Geometry check sheet. Reference: the model listing, model coordinates, mm. A direction names the side the tool comes from. Coordinates: 2 decimals unless noted, no trailing zeros. Order: outer loops, then holes, each group sorted by start corner. A loop starts at its lowest first (then second) coordinate and runs counter-clockwise, first axis right, second up. Notation, with made-up numbers: (34.5, -20) - (89.5, -20) arc R29 cw to (89.5, 5) - close; hole circle Ø11 at (5.5, -15). An arc over 180 degrees is marked (long way). Put each result on its own line as item: value.
from build123d import *

# Parameters (mm, degrees)
SKETCH1_R           = 5.1
SKETCH1_R_2         = 4.1
BOSS_EXTRUDE1_DEPTH = 5
SKETCH7_R           = 2.6
CUT_EXTRUDE1_DEPTH  = 7
BOSS_EXTRUDE7_DEPTH = 8
SKETCH9_R           = 1.5
CUT_EXTRUDE2_DEPTH  = 7
CUT_EXTRUDE3_DEPTH  = 10
SKETCH11_R          = 1
CUT_EXTRUDE4_DEPTH  = 10
CUT_EXTRUDE5_START  = 5
CUT_EXTRUDE5_DEPTH  = 5


with BuildPart() as part:
    # Sketch1 → Boss-Extrude1 (new body)
    with BuildSketch(Plane.XY):
        with BuildLine():
            Line((-58.265804598, 27.46480771), (50.206034483, 32.957769253))
            ThreePointArc((50.206034483, 32.957769253), (84.875, 0), (50.206034483, -32.957769253))
            Line((50.206034483, -32.957769253), (-58.265804598, -27.46480771))
            ThreePointArc((-58.265804598, -27.46480771), (-61.107119662, -27.172397082), (-63.902777778, -26.586845234))
            Line((-63.902777778, -26.586845234), (-105.963888889, -15.468709954))
            ThreePointArc((-105.963888889, -15.468709954), (-117.875, 0), (-105.963888889, 15.468709954))
            Line((-105.963888889, 15.468709954), (-63.902777778, 26.586845234))
            ThreePointArc((-63.902777778, 26.586845234), (-61.107119662, 27.172397082), (-58.265804598, 27.46480771))
        make_face()
        with Locations((51.875, 0)):
            Circle(SKETCH1_R, mode=Mode.SUBTRACT)
        with Locations((-101.875, 0)):
            Circle(SKETCH1_R_2, mode=Mode.SUBTRACT)
        with BuildLine():
            Line((-46.875, -18.2), (-56.875, -18.2))
            ThreePointArc((-56.875, -18.2), (-75.075, 0), (-56.875, 18.2))
            Line((-56.875, 18.2), (-46.875, 18.2))
            ThreePointArc((-46.875, 18.2), (-28.675, 0), (-46.875, -18.2))
        make_face(mode=Mode.SUBTRACT)
    extrude(amount=BOSS_EXTRUDE1_DEPTH)

    # Sketch7 → Cut-Extrude1 (cut)
    with BuildSketch(Plane.XY.offset(5)):
        with Locations((29.375, 0)):
            Circle(SKETCH7_R)
        with Locations((74.375, 0)):
            Circle(SKETCH7_R)
    extrude(amount=-CUT_EXTRUDE1_DEPTH, mode=Mode.SUBTRACT)

    # Sketch8 → Boss-Extrude7 (add)
    with BuildSketch(Plane.XY.offset(5)):
        Polygon((-28.993802154, 25), (-26.684401077, 21), (-22.065598923, 21), (-19.756197846, 25), (-22.065598923, 29), (-26.684401077, 29), align=None)
        Polygon((-25.775, 27.424871131), (-27.175, 25), (-25.775, 22.575128869), (-22.975, 22.575128869), (-21.575, 25), (-22.975, 27.424871131), align=None, mode=Mode.SUBTRACT)
    extrude(amount=-BOSS_EXTRUDE7_DEPTH)

    # Sketch9 → Cut-Extrude2 (cut)
    with BuildSketch(Plane.XY.offset(5)):
        with Locations((-24.375, 25)):
            Circle(SKETCH9_R)
    cut_extrude2 = extrude(amount=-CUT_EXTRUDE2_DEPTH, mode=Mode.SUBTRACT)

    # Mirror2: Cut-Extrude2 across plane
    add(cut_extrude2.mirror(Plane.ZX), mode=Mode.SUBTRACT)

    # Sketch10 → Cut-Extrude3 (cut)
    with BuildSketch(Plane.XY.offset(5)):
        with BuildLine():
            Line((-80.875, 17), (-74.875, 17))
            ThreePointArc((-74.875, 17), (-72.875, 15), (-74.875, 13))
            Line((-74.875, 13), (-80.875, 13))
            ThreePointArc((-80.875, 13), (-82.875, 15), (-80.875, 17))
        make_face()
        with BuildLine():
            Line((-22.875, 17), (-28.875, 17))
            ThreePointArc((-28.875, 17), (-30.875, 15), (-28.875, 13))
            Line((-28.875, 13), (-22.875, 13))
            ThreePointArc((-22.875, 13), (-20.875, 15), (-22.875, 17))
        make_face()
        with BuildLine():
            Line((-22.875, -17), (-28.875, -17))
            ThreePointArc((-28.875, -17), (-30.875, -15), (-28.875, -13))
            Line((-28.875, -13), (-22.875, -13))
            ThreePointArc((-22.875, -13), (-20.875, -15), (-22.875, -17))
        make_face()
        with BuildLine():
            Line((-80.875, -17), (-74.875, -17))
            ThreePointArc((-74.875, -17), (-72.875, -15), (-74.875, -13))
            Line((-74.875, -13), (-80.875, -13))
            ThreePointArc((-80.875, -13), (-82.875, -15), (-80.875, -17))
        make_face()
    extrude(amount=-CUT_EXTRUDE3_DEPTH, mode=Mode.SUBTRACT)

    # Sketch11 → Cut-Extrude4 (cut)
    with BuildSketch(Plane.XY.offset(5)):
        with Locations((-115.168208365, -3.514699328)):
            Circle(SKETCH11_R)
        with Locations((-88.581791635, 3.514699328)):
            Circle(SKETCH11_R)
    extrude(amount=-CUT_EXTRUDE4_DEPTH, mode=Mode.SUBTRACT)

    # Sketch12 → Cut-Extrude5 (cut)
    with BuildSketch(Plane(origin=(0, 0, 0), x_dir=(-1, 0, 0), z_dir=(0, 0, -1)).offset(CUT_EXTRUDE5_START)):
        with BuildLine():
            Line((105.963888889, 15.468709954), (63.902777778, 26.586845234))
            ThreePointArc((63.902777778, 26.586845234), (61.107119662, 27.172397082), (58.265804598, 27.46480771))
            Line((58.265804598, 27.46480771), (-50.206034483, 32.957769253))
            ThreePointArc((-50.206034483, 32.957769253), (-84.875, 0), (-50.206034483, -32.957769253))
            Line((-50.206034483, -32.957769253), (58.265804598, -27.46480771))
            ThreePointArc((58.265804598, -27.46480771), (61.107119662, -27.172397082), (63.902777778, -26.586845234))
            Line((63.902777778, -26.586845234), (105.963888889, -15.468709954))
            ThreePointArc((105.963888889, -15.468709954), (117.875, 0), (105.963888889, 15.468709954))
        make_face()
    extrude(amount=-CUT_EXTRUDE5_DEPTH, mode=Mode.SUBTRACT)


solid = part.part
Q1. Section check C-C on x = 23.5. Record the boundary of the cut face in (y, z).
Answer block:
outline: (-31.61, 0) - (31.61, 0) - (31.61, 5) - (-31.61, 5) - close
Q2. Access from +Z, -Z, +X, -X, +Y, -Y to the whole of each face (thin tool, end or side, straight path). Record for faces 1 (the flat face through (-3.27, -30.25, 2.46)), 2 (the flat face through (-78, 17, 3)).
Answer block:
face 1: +Z, -Z, -X, -Y
face 2: +Z, -Z
Q3. Draft check along Y on faces 3 (the flat face through (7, 0, 0)), 4 (the flat face through (-78, -17, 3)), 5 (the cylindrical face through (-61.07, -27.18, 2.46)). Enter one of: pulls with the +Y half, pulls with the -Y half, needs draft (parallel to the pull), parting line crosses it, or undercut.
Answer block:
face 3: needs draft
face 4: undercut
face 5: pulls with the -Y half
Q4. Section check B-B on z = 1.4. State how many separate pieces and enclosed holes the cut face has, then the cut area to 3 significant figures.
Answer block:
separate pieces: 1
enclosed holes: 13
area: 8,970 mm^2
Q5. Section check A-A on y = 0. Record the boundary of the cut face in (x, z) (3 decimals).
Answer block:
outline: (-117.875, 0) - (-105.975, 0) - (-105.975, 5) - (-117.875, 5) - close; (-97.775, 0) - (-75.075, 0) - (-75.075, 5) - (-97.775, 5) - close; (-28.675, 0) - (26.775, 0) - (26.775, 5) - (-28.675, 5) - close; (31.975, 0) - (46.775, 0) - (46.775, 5) - (31.975, 5) - close; (56.975, 0) - (71.775, 0) - (71.775, 5) - (56.975, 5) - close; (76.975, 0) - (84.875, 0) - (84.875, 5) - (76.975, 5) - close
Q6. Depth check by flat-ended pin: pin 1 Ø2.5 at (x, y) = (-24.375, -25) entering from +Z; pin 2 Ø2.5 at (x, z) = (-52.5, 2) entering from +Y; pin 3 Ø2.5 at (x, z) = (-25.5, 3) entering from +Y; pin 4 Ø1.5 at (x, z) = (-77.5, 3) entering from -Y. Enter the tip coordinate at first touch or a pass-through.
Answer block:
pin 1: passes through
pin 2: stops at y = 27.82
pin 3: stops at y = 29.19
pin 4: stops at y = -23.19
Q7. Thickness scan on L1, parallel to Y at x = -79, z = 2.2; L2, parallel to X at y = -10, z = 4.45 (3 decimals); L3, parallel to Y at x = 54.5, z = 2.9. Record the ranges inside material, lowest first. Write a range as [from, to].
Answer block:
L1: y = [-22.6, -17], [-13, 13], [17, 22.6]
L2: x = [-114.365, -72.082], [-31.668, 83.323]
L3: y = [-32.9, -4.37], [4.37, 32.9]
